CAD build for the part. Positions are in the model's coordinates, mm. Round coordinates to 2 decimals unless told otherwise and drop trailing zeros. Order: outer loops, then holes, each group sorted by start corner. A loop starts at its lowest first (then second) coordinate and runs counter-clockwise, first axis right, second up.
Autodesk Fusion 360 part; units mm, degrees
sketch "Skizze1" plane through (0, 0, 0) normal (0, 1, 0) x (1, 0, 0)
  line L0 (0, 0) -> (94, 0)
  line L1 (0, 0) -> (0, -19)
  line L2 (0, -19) -> (94, -19)
  line L3 (94, -19) -> (94, 0)
  dimension "d1" = 94
  dimension "d2" = 19
extrude "Extrusion1" add sketch "Skizze1" along normal blind 2
sketch "Skizze2" plane through (0, 0, 0) normal (0, -1, 0) x (1, 0, 0)
  line L0 (0, 19) -> (0, 0)
  line L1 (0, 0) -> (94, 0)
  line L2 (94, 0) -> (94, 19)
  line L3 (94, 19) -> (0, 19)
  circle A0 centre (3.75, 9.5) radius 1.75
  circle A1 centre (90.25, 9.5) radius 1.75
  dimension "d8" = 3.5
  dimension "d9" = 3.5
extrude "Extrusion2" cut sketch "Skizze2" against normal blind 2 contours A0 | A1
fillet "Abrundung1" radius 2 4 edges at (47, 0, 19) (94, 0, 9.5) (47, 0, 0) (0, 0, 9.5)
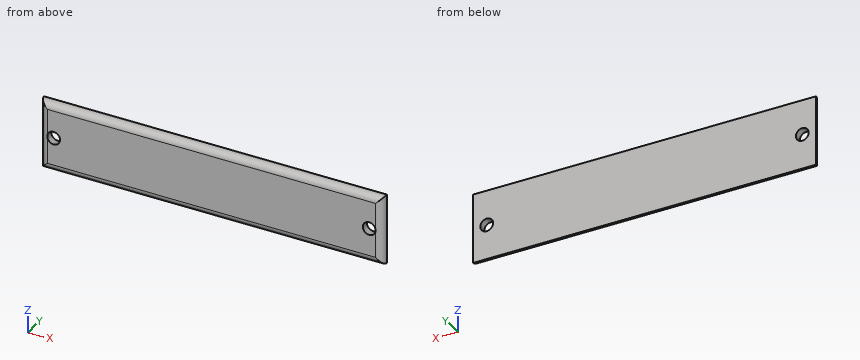
1. Cut at A-A, the plane z = 9.5. Give the number of separate pieces and of enclosed holes in the cut face, and give its area (3 significant figures).
2. Drill centre lines: line 1 (X direction, y = 1.8, z = 10.75); line 2 (Z direction, x = 90.25, y = 0.7); line 3 (Z direction, x = 3.75, y = 1.3). Where is each one in solid material? Low to high.
3. Cut at C-C, the plane y = 0.9. Write the cut outline in (x, z).
Outcome:
1. separate pieces: 3
1. enclosed holes: 0
1. area: 172 mm2
2. line 1: x = 0.01 to 2.53, 4.97 to 89.03, 91.47 to 93.99
2. line 2: z = 0.48 to 7.75, 11.25 to 18.52
2. line 3: z = 0.13 to 7.75, 11.25 to 18.87
3. outline: (0.33, 0.33) - (93.67, 0.33) - (93.67, 18.67) - (0.33, 18.67) - close; hole circle Ø3.5 at (3.75, 9.5); hole circle Ø3.5 at (90.25, 9.5)
